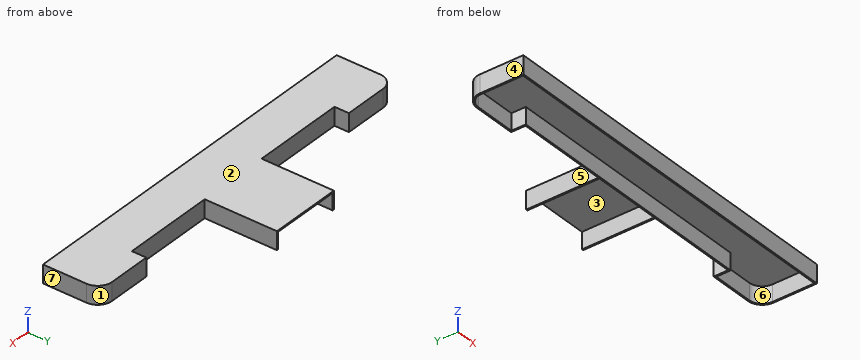
```python
from build123d import *

# Parameters (mm, degrees)
BOSS_EXTRUDE1_DEPTH = 25
SKETCH2_W           = 96
SKETCH2_H           = 23
CUT_EXTRUDE1_DEPTH  = 100
SHELL3_START        = -25
SHELL3_DEPTH        = 23


# Read off the part's stored shape, not the designer's step: Shell3
with BuildPart() as part:
    # Sketch1 → Boss-Extrude1 (new body)
    with BuildSketch(Plane.XY):
        with BuildLine():
            Line((0, 0), (516, 0))
            Line((516, 0), (516, 60))
            ThreePointArc((516, 60), (510.142135624, 74.142135624), (496, 80))
            Line((496, 80), (436, 80))
            Line((436, 80), (436, 60))
            Line((436, 60), (308, 60))
            Line((308, 60), (308, 160))
            Line((308, 160), (208, 160))
            Line((208, 160), (208, 60))
            Line((208, 60), (80, 60))
            Line((80, 60), (80, 80))
            Line((80, 80), (20, 80))
            ThreePointArc((20, 80), (5.857864376, 74.142135624), (0, 60))
            Line((0, 60), (0, 0))
        make_face()
    extrude(amount=-BOSS_EXTRUDE1_DEPTH)

    # Sketch2 → Cut-Extrude1 (cut)
    with BuildSketch(Plane(origin=(0, 160, 0), x_dir=(1, 0, 0), z_dir=(0, 1, 0))):
        with Locations((258, 13.5)):
            Rectangle(SKETCH2_W, SKETCH2_H)
    extrude(amount=-CUT_EXTRUDE1_DEPTH, mode=Mode.SUBTRACT)

    # Shell3 outline → Shell3 (cut)
    with BuildSketch(Plane.XY.offset(SHELL3_START)):
        with BuildLine():
            ThreePointArc((20, 78), (7.272077939, 72.727922061), (2, 60))
            Line((2, 60), (2, 2))
            Line((2, 2), (514, 2))
            Line((514, 2), (514, 60))
            ThreePointArc((514, 60), (508.727922061, 72.727922061), (496, 78))
            Line((496, 78), (438, 78))
            Line((438, 78), (438, 58))
            Line((438, 58), (78, 58))
            Line((78, 58), (78, 78))
            Line((78, 78), (20, 78))
        make_face()
    extrude(amount=SHELL3_DEPTH, mode=Mode.SUBTRACT)


solid = part.part
```
Input: part model. Units: mm. Frame: model coordinates. Face numbers are marked on the shaded views. A direction names the side the tool comes from. Give positions to 0.01 mm unless a question says otherwise; leave off trailing zeros. Order: outer loops, then holes, each group sorted by start corner. A loop starts at its lowest first (then second) coordinate and runs counter-clockwise, first axis right, second up.
1. Mould query, pull axis X, two halves, no side actions, for the marked faces 1, 2, 3 and 4. Classes: released by +X, released by -X, zero draft, split by the parting line, or undercut.
Derived:
face 1: released by +X
face 2: zero draft
face 3: undercut
face 4: released by -X
2. Pin query (flat end, axial travel): pin 1 (2 mm diameter, centred on y = 138, z = -5, fed in from -X); pin 2 (1.5 mm diameter, centred on x = 338, z = -4.5, fed in from +Y); pin 3 (6 mm diameter, centred on y = 68, z = -17, fed in from -X). Return the tip coordinate at first contact, or that it passes through.
Derived:
pin 1: stops at x = 208
pin 2: stops at y = 60
pin 3: stops at x = 0.64
3. Section A-A on z = -10.5. Return the cut outline in (x, y), and give its area (3 significant figures).
Derived:
outline: (0, 0) - (516, 0) - (516, 60) arc R20 ccw to (496, 80) - (436, 80) - (436, 60) - (308, 60) - (308, 160) - (306, 160) - (306, 60) - (210, 60) - (210, 160) - (208, 160) - (208, 60) - (80, 60) - (80, 80) - (20, 80) arc R20 ccw to (0, 60) - close; hole (2, 2) - (514, 2) - (514, 60) arc R18 ccw to (496, 78) - (438, 78) - (438, 58) - (78, 58) - (78, 78) - (20, 78) arc R18 ccw to (2, 60) - close
area: 2,820 mm2
4. Reachability of the marked faces 5, 6 and 7 from +Z, -Z, +X, -X, +Y, -Y: full face, straight path, thin tool, end or side. Return the list, or none.
Derived:
face 5: +Z, -Z, +Y
face 6: -Z
face 7: +Z, -Z, +X, +Y, -Y
5. Section C-C on y = 27.5. Return the cut outline in (x, z).
Derived:
outline: (0, -25) - (2, -25) - (2, -2) - (514, -2) - (514, -25) - (516, -25) - (516, 0) - (0, 0) - close
6. Section B-B on x = 221. Return the cut outline in (y, z).
Derived:
outline: (0, -25) - (2, -25) - (2, -2) - (58, -2) - (58, -25) - (60, -25) - (60, -2) - (160, -2) - (160, 0) - (0, 0) - close
7. Material intervals for L1, parallel to X at y = 49, z = -6; L2, parallel to Y at x = 238, z = -19; L3, parallel to X at y = 68.5, z = -11, sorted ascending.
Derived:
L1: x = 0 to 2, 514 to 516
L2: y = 0 to 2, 58 to 60
L3: x = 1.9 to 4.13, 78 to 80, 208 to 210, 306 to 308, 436 to 438, 511.87 to 514.1
8. Section D-D on x = 135. Return the cut outline in (y, z), and give its area (3 significant figures).
Derived:
outline: (0, -25) - (2, -25) - (2, -2) - (58, -2) - (58, -25) - (60, -25) - (60, 0) - (0, 0) - close
area: 212 mm2
